```python
from build123d import *

# Parameters (mm, degrees)
SKETCH003_W     = 5
SKETCH003_H     = 25
SKETCH003_R     = 1.5
PAD001_DEPTH    = 5
SKETCH004_W     = 5
SKETCH004_H     = 5
POCKET002_DEPTH = 4
CHAMFER003_SIZE = 1.5
CHAMFER004_SIZE = 2
CHAMFER005_SIZE = 1


with BuildPart() as part:
    # Sketch003 (on DatumPlane) → Pad001 (new body)
    with BuildSketch(Plane(origin=(0, 0, 0), x_dir=(0, 0, -1), z_dir=(-1, 0, 0))):
        with Locations((-10, 20)):
            Rectangle(SKETCH003_W, SKETCH003_H)
        with Locations((-10, 30)):
            Circle(SKETCH003_R, mode=Mode.SUBTRACT)
        with Locations((-10, 10)):
            Circle(SKETCH003_R, mode=Mode.SUBTRACT)
    extrude(amount=PAD001_DEPTH)

    # Sketch004 (on Face8 of Pad001) → Pocket002 (cut)
    with BuildSketch(Plane(origin=(-5, 0, 0), x_dir=(0, 0, -1), z_dir=(-1, 0, 0))):
        with Locations((-10, 30)):
            Rectangle(SKETCH004_W, SKETCH004_H)
        with Locations((-10, 10)):
            Rectangle(SKETCH004_W, SKETCH004_H)
    extrude(amount=-POCKET002_DEPTH, mode=Mode.SUBTRACT)

    # Chamfer003
    chamfer003_edges = [part.edges().sort_by_distance(p)[0] for p in [
        (-5, -20, 12.5),
        (-5, -20, 7.5),
    ]]
    chamfer(chamfer003_edges, length=CHAMFER003_SIZE)

    # Chamfer004
    chamfer004_edges = [part.edges().sort_by_distance(p)[0] for p in [
        (-5, -12.5, 10),
        (-5, -27.5, 10),
    ]]
    chamfer(chamfer004_edges, length=CHAMFER004_SIZE)

    # Chamfer005
    chamfer005_edges = [part.edges().sort_by_distance(p)[0] for p in [
        (-0.5, -7.5, 7.5),
        (-0.5, -7.5, 12.5),
        (-0.5, -32.5, 7.5),
        (-0.5, -32.5, 12.5),
    ]]
    chamfer(chamfer005_edges, length=CHAMFER005_SIZE)


solid = part.part
```
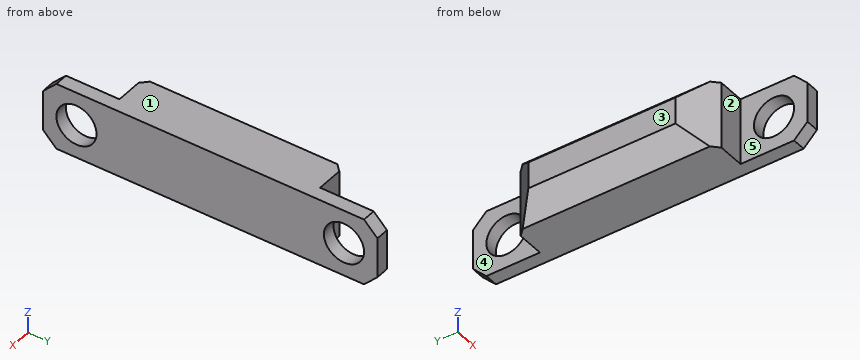
Part model, mm, in its own coordinate system. Face numbers are marked on the shaded views. A direction names the side the tool comes from. Round coordinates to 2 decimals unless told otherwise and drop trailing zeros. Loops run counter-clockwise (first coordinate to the right, second up) from the corner with the lowest first, then second, coordinate; pieces in that order, holes last.
1. Slice it at D-D (y = -14.75). Give the cut face in (x, z), and give its area (4 significant figures).
Solutions:
outline: (-5, 9) - (-3.5, 7.5) - (0, 7.5) - (0, 12.5) - (-3.5, 12.5) - (-5, 11) - close
area: 22.75 mm2
2. Two-plate mould, pull along Y, no slides. Class the marked faces 1 and 2: pulls with the +Y half, pulls with the -Y half, needs draft (parallel to the pull), parting line crosses it, or undercut.
Solutions:
face 1: needs draft
face 2: pulls with the -Y half
3. Slice it at A-A (z = 10). Give the cut face in (x, y), and give its area (3 significant figures).
Solutions:
outline: (-5, -25.5) - (-3, -27.5) - (-1, -27.5) - (-1, -28.5) - (0, -28.5) - (0, -11.5) - (-1, -11.5) - (-1, -12.5) - (-3, -12.5) - (-5, -14.5) - close; (-1, -32.5) - (0, -32.5) - (0, -31.5) - (-1, -31.5) - close; (-1, -8.5) - (0, -8.5) - (0, -7.5) - (-1, -7.5) - close
area: 75.0 mm2
4. Slice it at B-B (y = -30). Give the cut face in (x, z).
Solutions:
outline: (-1, 7.5) - (0, 7.5) - (0, 8.5) - (-1, 8.5) - close; (-1, 11.5) - (0, 11.5) - (0, 12.5) - (-1, 12.5) - close
5. Slice it at C-C (z = 8.1). Give the cut face in (x, y), and give its area (3 significant figures).
Solutions:
outline: (-4.1, -26.4) - (-3, -27.5) - (-1, -27.5) - (-1, -32.1) - (0, -32.1) - (0, -7.9) - (-1, -7.9) - (-1, -12.5) - (-3, -12.5) - (-4.1, -13.6) - close
area: 69.5 mm2
6. Drill centre lines: line 1 along Y through (x, z) = (-0.25, 10); line 2 along Z through (x, y) = (-0.3, -30); line 3 along Y through (x, z) = (-2.5, 11.2). Where is each one in solid material? Low to high.
Solutions:
line 1: y = -32.5 to -31.5, -28.5 to -11.5, -8.5 to -7.5
line 2: z = 7.5 to 8.5, 11.5 to 12.5
line 3: y = -27.5 to -12.5
7. 3-axis set-ups, long thin cutter, end or side, ignore diameter. For the marked faces 3, 4 and 5: which of +Z, -Z, +X, -X, +Y, -Y reach the whole face in a straight line?
Solutions:
face 3: +Z, -Z, -X, +Y, -Y
face 4: +Z, -Z, -X, +Y
face 5: +Z, -Z, -X, -Y
8. Flat gauge pins, fed straight in: pin 1 (0.6 mm diameter, centred on x = -2, z = 11, fed in from -Y); pin 2 (3 mm diameter, centred on y = -28, z = 11.5, fed in from +X); pin 3 (2.5 mm diameter, centred on y = -10, z = 10, fed in from -X). Where does each tip first touch, or does it go through?
Solutions:
pin 1: stops at y = -27.5
pin 2: stops at x = 0
pin 3: passes through
